CAD build for the part. Positions are in the model's coordinates, mm. A direction names the side the tool comes from. Give positions to 0.01 mm unless a question says otherwise; leave off trailing zeros. Loops run counter-clockwise (first coordinate to the right, second up) from the corner with the lowest first, then second, coordinate; pieces in that order, holes last. Notation, with made-up numbers: M 34,-37.5 L 55,-37.5 A19 cw 55,-30.5 Z; hole C -17,24.5 d7. An arc over 180 degrees is marked long. Answer as CSV lines item,"result".
from build123d import *

# Parameters (mm, degrees)
F1_DEPTH     = 80
F2_T         = 4
F3_T1_DEPTH  = 774.9998275448
F3_T3_DEPTH  = 124.9996550895
F3_T6_ANGLE  = 90.0000000944
F3_T8_ANGLE  = 89.9999999363
F3_T10_ANGLE = 90.0000000944
F3_T12_ANGLE = 89.9999999363
F4_R         = 15
F5_DEPTH     = 80.001


# Not quite as in the source:
# - a fillet or chamfer that OpenCascade refuses, or shapes differently, is made with other operations: its cross-section is extruded or revolved along the edge and cut away or added
# - a shell that OpenCascade refuses in one call is made with other operations: the cavity is built on its own and cut out


with BuildPart() as f1:
    # F0 (on Front) → F1 (new body)
    with BuildSketch(Plane.XZ):
        with BuildLine():
            Line((-374.9998275448, -50), (375, -50))
            Line((375, -50), (375, 50))
            Line((375, 50), (-374.9998275448, 50))
            ThreePointArc((-374.9998275448, 50), (-374.999949489, 49.999949489), (-375, 49.9998275448))
            Line((-375, 49.9998275448), (-375, -49.9998275448))
            ThreePointArc((-375, -49.9998275448), (-374.999949489, -49.999949489), (-374.9998275448, -50))
        make_face()
    extrude(amount=F1_DEPTH)

    # F2: shell of thickness 4, made by hand


with BuildPart() as f2_core1:
    # F2_t2: copy of F1
    add(f1.part)

    # the walls: a layer under each face that stays
    f2_faces = [f2_core1.faces().sort_by_distance(p)[0] for p in [
        (8.62276e-05, -40, -50),
        (8.62276e-05, -40, 50),
        (0, 0, 0),
        (0, -80, 0),
    ]]
    thicken(f2_faces, amount=-F2_T, mode=Mode.SUBTRACT)


with BuildPart() as f1_1:
    add(f1.part)

    # what is left inside the walls is the cavity
    f2_cavity = [f2_core1.part.solids().sort_by_distance(p)[0] for p in [
        (0, -4.04, -16.666667),
    ]]
    add(f2_cavity, mode=Mode.SUBTRACT)

    # F3: fillet of radius 5 on 4 edges, made by hand

    # F3_s2 → F3_t1 (cut)
    with BuildSketch(Plane.YZ.offset(-387.4998275448)):
        with BuildLine():
            ThreePointArc((-80, 45), (-78.5355339059, 48.5355339059), (-75, 50))
            Line((-75, 50), (-80, 50))
            Line((-80, 50), (-80, 45))
        make_face()
        with BuildLine():
            ThreePointArc((0, 45), (-1.4644660941, 48.5355339059), (-5, 50))
            Line((-5, 50), (0, 50))
            Line((0, 50), (0, 45))
        make_face()
        with BuildLine():
            ThreePointArc((-5, -50), (-1.4644660941, -48.5355339059), (0, -45))
            Line((0, -45), (0, -50))
            Line((0, -50), (-5, -50))
        make_face()
        with BuildLine():
            ThreePointArc((-75, -50), (-78.5355339059, -48.5355339059), (-80, -45))
            Line((-80, -45), (-80, -50))
            Line((-80, -50), (-75, -50))
        make_face()
    extrude(amount=F3_T1_DEPTH, mode=Mode.SUBTRACT)

    # F3_s4 → F3_t3 (cut)
    with BuildSketch(Plane.XY.offset(-62.4998275448)):
        with BuildLine():
            ThreePointArc((-370, -80), (-373.5355339059, -78.5355339059), (-375, -75))
            Line((-375, -75), (-375, -80))
            Line((-375, -80), (-370, -80))
        make_face()
        with BuildLine():
            ThreePointArc((-370, 0), (-373.5355339059, -1.4644660941), (-375, -5))
            Line((-375, -5), (-375, 0))
            Line((-375, 0), (-370, 0))
        make_face()
    extrude(amount=F3_T3_DEPTH, mode=Mode.SUBTRACT)

    # F3_s5 → F3_t6 (revolve, cut)
    with BuildSketch(Plane.XY.offset(-49.9998275448)):
        with BuildLine():
            ThreePointArc((-375, -75), (-374.999956886, -75.0207638646), (-374.9998275448, -75.0415273711))
            Line((-374.9998275448, -75.0415273711), (-374.9998275448, -80))
            Line((-374.9998275448, -80), (-375, -80))
            Line((-375, -80), (-375, -75))
        make_face()
    revolve(axis=Axis((-374.9998275448, -80, -49.9998275448), (0, -1, 0)), revolution_arc=F3_T6_ANGLE, mode=Mode.SUBTRACT)

    # F3_s7 → F3_t8 (revolve, cut)
    with BuildSketch(Plane.YZ.offset(-374.9998275448)):
        with BuildLine():
            ThreePointArc((-75.0415273711, 49.9998275448), (-75.0207638646, 49.999956886), (-75, 50))
            Line((-75, 50), (-80, 50))
            Line((-80, 50), (-80, 49.9998275448))
            Line((-80, 49.9998275448), (-75.0415273711, 49.9998275448))
        make_face()
    revolve(axis=Axis((-374.9998275448, -80, 49.9998275448), (0, -1, 0)), revolution_arc=F3_T8_ANGLE, mode=Mode.SUBTRACT)

    # F3_s9 → F3_t10 (revolve, cut)
    with BuildSketch(Plane.XY.offset(-49.9998275448)):
        with BuildLine():
            ThreePointArc((-375, -5), (-374.999956886, -4.9792361354), (-374.9998275448, -4.9584726289))
            Line((-374.9998275448, -4.9584726289), (-374.9998275448, 0))
            Line((-374.9998275448, 0), (-375, 0))
            Line((-375, 0), (-375, -5))
        make_face()
    revolve(axis=Axis((-374.9998275448, 0, -49.9998275448), (0, -1, 0)), revolution_arc=F3_T10_ANGLE, mode=Mode.SUBTRACT)

    # F3_s11 → F3_t12 (revolve, cut)
    with BuildSketch(Plane.YZ.offset(-374.9998275448)):
        with BuildLine():
            ThreePointArc((-4.9584726289, 49.9998275448), (-4.9792361354, 49.999956886), (-5, 50))
            Line((-5, 50), (0, 50))
            Line((0, 50), (0, 49.9998275448))
            Line((0, 49.9998275448), (-4.9584726289, 49.9998275448))
        make_face()
    revolve(axis=Axis((-374.9998275448, 0, 49.9998275448), (0, -1, 0)), revolution_arc=F3_T12_ANGLE, mode=Mode.SUBTRACT)

    # F4 (on Front) → F5 (cut, through all)
    with BuildSketch(Plane.XZ):
        with Locations((302, -10)):
            Circle(F4_R)
    extrude(amount=F5_DEPTH, mode=Mode.SUBTRACT)


solid = f1_1.part
1) Mould opens along Z. For faces 1 (the face through (315.856, -1.972, -15.745)), 2 (the face through (5, -40, 50)), 3 (the face through (315.856, -77.972, -15.745)), 4 (the face through (-3, 0, 1)) say: +Z half, -Z half, draft (parallel to the pull), parting line (faces both ways), or undercut.
Answer below:
face 1,"undercut"
face 2,"+Z half"
face 3,"undercut"
face 4,"draft"
2) Band-saw the part on C-C on y = -21.5. Give the cut face in (x, z).
Answer below:
outline,"M -375,-50 L 375,-50 L 375,-46 L -375,-46 Z; M -375,46 L 375,46 L 375,50 L -375,50 Z"
3) Band-saw the part on D-D on x = 302. Give the cut face in (y, z), and give its area (3 significant figures).
Answer below:
outline,"M -80,-45 A5 ccw -75,-50 L -5,-50 A5 ccw 0,-45 L 0,-25 L -4,-25 L -4,-46 L -76,-46 L -76,-25 L -80,-25 Z; M -80,5 L -76,5 L -76,46 L -4,46 L -4,5 L 0,5 L 0,45 A5 ccw -5,50 L -75,50 A5 ccw -80,45 Z"
area,"1,110 mm^2"
4) Band-saw the part on A-A on x = 129.5. Give the cut face in (y, z), and give its area (3 significant figures).
Answer below:
outline,"M -80,-45 A5 ccw -75,-50 L -5,-50 A5 ccw 0,-45 L 0,45 A5 ccw -5,50 L -75,50 A5 ccw -80,45 Z; hole M -76,-46 L -4,-46 L -4,46 L -76,46 Z"
area,"1,350 mm^2"
5) Which spindle directions (+Z, -Z, +X, -X, +Y, -Y) get a long thin tool onto all of the face, cutting with end or side? Do faces 5 (the face through (5, -39, 46)), 6 (the face through (-3, -80, 1)). Say none if no direction does.
Answer below:
face 5,"+X, -X"
face 6,"+Z, -Z, +X, -X, -Y"
6) Drill centre lines: line 1 (Z direction, x = 328, y = -49.5); line 2 (Y direction, x = 311.5, z = -22.5); line 3 (Z direction, x = 302, y = -78.95). Where is each one in solid material? Low to high. Write a range as from..to.
Answer below:
line 1,"z = -50..-46, 46..50"
line 2,"y = -80..-76, -4..0"
line 3,"z = -48.07..-25, 5..48.07"
7) Band-saw the part on B-B on z = -10. Give the cut face in (x, y).
Answer below:
outline,"M -374.9,-76 A5 ccw -370,-80 L 287,-80 L 287,-76 Z; M -374.9,-4 L 287,-4 L 287,0 L -370,0 A5 ccw Z; M 317,-80 L 375,-80 L 375,-76 L 317,-76 Z; M 317,-4 L 375,-4 L 375,0 L 317,0 Z"
8) Flat gauge pin, fed straight in: pin 1 (24 mm diameter, centred on x = 302, z = -10, fed in from +Y). Where does the tip first touch, or does it go through?
Answer below:
pin 1,"passes through"
